Design review of the part built by this model. Coordinates are the model's own, in mm. A direction names the side the tool comes from. Give positions to 0.01 mm unless a question says otherwise; leave off trailing zeros. Write each loop counter-clockwise with the first axis right and the second up, starting at its lowest first coordinate (ties: lowest second). Pieces come first, ordered by that corner, then holes. Notation, with made-up numbers: (-30.75, 26.5) - (-5.75, 26.5) arc R14 cw to (-5.75, 47.5) - close; hole circle Ø11 at (-34.75, 27). An arc over 180 degrees is marked (long way). Write each question's results on one line, items separated by ' | '. Start each with the question number.
from build123d import *

# Parameters (mm, degrees)
SKETCH1_W                 = 26.4
SKETCH1_H                 = 26.4
BOSS_EXTRUDE1_DEPTH       = 26.2
FILLET1_R                 = 2.032
SKETCH5_R                 = 12.626192159
CUT_EXTRUDE3_DEPTH        = 2.5
M2X0_4_TAPPED_HOLE1_D     = 1.6
M2X0_4_TAPPED_HOLE1_DEPTH = 5.334
M2X0_4_TAPPED_HOLE2_D     = 1.6
M2X0_4_TAPPED_HOLE2_DEPTH = 5.334


with BuildPart() as part:
    # Sketch1 → Boss-Extrude1 (new body)
    with BuildSketch(Plane.XY):
        Rectangle(SKETCH1_W, SKETCH1_H)
    extrude(amount=BOSS_EXTRUDE1_DEPTH)

    # Fillet1
    fillet1_edges = [part.edges().sort_by_distance(p)[0] for p in [
        (-13.2, 13.2, 13.1),
        (13.2, 13.2, 13.1),
        (13.2, -13.2, 13.1),
        (-13.2, -13.2, 13.1),
    ]]
    fillet(fillet1_edges, radius=FILLET1_R)

    # Sketch5 → Cut-Extrude3 (cut)
    with BuildSketch(Plane(origin=(0, 0, 0), x_dir=(-1, 0, 0), z_dir=(0, 0, -1))):
        Circle(SKETCH5_R)
    extrude(amount=-CUT_EXTRUDE3_DEPTH, mode=Mode.SUBTRACT)

    # M2x0.4 Tapped Hole1
    with Locations(Plane(origin=(0, -13.2, 0), x_dir=(-1, 0, 0), z_dir=(0, -1, 0))):
        with Locations((9, -23.5), (9, -5.5), (-9, -5.5), (-9, -23.5)):
            Hole(M2X0_4_TAPPED_HOLE1_D / 2, depth=M2X0_4_TAPPED_HOLE1_DEPTH)

    # M2x0.4 Tapped Hole2
    with Locations(Plane(origin=(0, 13.2, 0), x_dir=(1, 0, 0), z_dir=(0, 1, 0))):
        with Locations((9, -5.5), (9, -23.5), (-9, -23.5), (-9, -5.5)):
            Hole(M2X0_4_TAPPED_HOLE2_D / 2, depth=M2X0_4_TAPPED_HOLE2_DEPTH)


solid = part.part
Q1. The part is to be moulded in two halves that separate along X. For faces 1 (the face through (-9.63, -10.5, 5.99)), 2 (the face through (-12.62, 12.59, 13.28)), 3 (the face through (9, 7.866, 23)), 4 (the face through (0, 0, 26.2)), say which applies: +X half, -X half, draft (parallel to the pull), parting line (faces both ways), or undercut.
Q2. Insertion check: P1, Ø0.5, axis at x = 9, z = 5.5, coming from the +Y side; P2, Ø1, axis at x = 9, z = 23.5, coming from the -Y side; P3, Ø2, axis at x = -9, z = 23.5, coming from the -Y side; P4, Ø7.5, axis at x = -3, y = 0.5, coming from the -Z side. Each pin has a flat end and moves straight along its axis. Give the tip position at first contact, or say it passes through.
Q3. For line 1 along Z through (x, y) = (-9, -9.25); line 2 along X through (y, z) = (-9.2, 5.5); line 3 along Y through (x, z) = (0, 1.5), list the stretches that pass through material, from the lowest coordinate up. Write a range as [from, to].
Q4. Machinability: for faces 5 (the face through (-9, -7.866, 5)), 6 (the face through (0, 0, 2.5)), 7 (the face through (9, 7.866, 5)), which of the approach directions +Z, -Z, +X, -X, +Y, -Y give a long, thin tool a straight path to every point of the face, cutting with its end or side? Answer none if there is none.
Q5. Add section B-B on y = 8.75. State the section outline as (x, z) points.
Q6. Add section D-D on y = 0. State the section outline as (x, z) points, plus the area to 3 significant figures.
Q7. Add section A-A on z = 23.5. State the section outline as (x, y) points.
Q8. Add section C-C on x = -5. State the section outline as (y, z) points.
Result:
1) face 1: undercut | face 2: -X half | face 3: undercut | face 4: draft
2) P1: stops at y = 7.87 | P2: stops at y = -7.87 | P3: stops at y = -13.2 | P4: stops at z = 2.5
3) line 1: z = [0, 4.7], [6.3, 22.7], [24.3, 26.2] | line 2: x = [-13.2, -9.8], [-8.2, 8.2], [9.8, 13.2] | line 3: y = [-13.2, -12.63], [12.63, 13.2]
4) face 5: -Y | face 6: -Z | face 7: +Y
5) outline: (-13.2, 0) - (-9.1, 0) - (-9.1, 2.5) - (9.1, 2.5) - (9.1, 0) - (13.2, 0) - (13.2, 26.2) - (-13.2, 26.2) - close; hole circle Ø1.6 at (-9, 5.5); hole circle Ø1.6 at (-9, 23.5); hole circle Ø1.6 at (9, 5.5); hole circle Ø1.6 at (9, 23.5)
6) outline: (-13.2, 0) - (-12.63, 0) - (-12.63, 2.5) - (12.63, 2.5) - (12.63, 0) - (13.2, 0) - (13.2, 26.2) - (-13.2, 26.2) - close | area: 629 mm²
7) outline: (-13.2, -11.17) arc R2.03 ccw to (-11.17, -13.2) - (-9.8, -13.2) - (-9.8, -7.87) - (-8.2, -7.87) - (-8.2, -13.2) - (8.2, -13.2) - (8.2, -7.87) - (9.8, -7.87) - (9.8, -13.2) - (11.17, -13.2) arc R2.03 ccw to (13.2, -11.17) - (13.2, 11.17) arc R2.03 ccw to (11.17, 13.2) - (9.8, 13.2) - (9.8, 7.87) - (8.2, 7.87) - (8.2, 13.2) - (-8.2, 13.2) - (-8.2, 7.87) - (-9.8, 7.87) - (-9.8, 13.2) - (-11.17, 13.2) arc R2.03 ccw to (-13.2, 11.17) - close
8) outline: (-13.2, 0) - (-11.59, 0) - (-11.59, 2.5) - (11.59, 2.5) - (11.59, 0) - (13.2, 0) - (13.2, 26.2) - (-13.2, 26.2) - close
